from build123d import *

# Parameters (mm, degrees)
F0_W     = 50.8
F0_H     = 54.61
F0_R     = 1.5875
F1_DEPTH = 50.8
F2_R     = 3.96875
F3_DEPTH = 54.611
F4_W     = 50.8
F4_H     = 50.546
F5_DEPTH = 33.9065
F6_W     = 11.43125
F6_H     = 2.032
F7_DEPTH = 2.033


with BuildPart() as f1:
    # F0 (on Front) → F1 (new body)
    with BuildSketch(Plane.XZ):
        Rectangle(F0_W, F0_H)
        with Locations((-9.525, -19.05)):
            Circle(F0_R, mode=Mode.SUBTRACT)
        with Locations((9.525, -19.05)):
            Circle(F0_R, mode=Mode.SUBTRACT)
        with Locations((-9.525, 19.05)):
            Circle(F0_R, mode=Mode.SUBTRACT)
        with Locations((9.525, 19.05)):
            Circle(F0_R, mode=Mode.SUBTRACT)
    extrude(amount=F1_DEPTH)

    # F2 (on face) → F3 (cut, through all)
    with BuildSketch(Plane.XY.offset(27.305)):
        with BuildLine():
            Line((-25.4, -2.032), (-25.4, -50.8))
            Line((-25.4, -50.8), (25.4, -50.8))
            Line((25.4, -50.8), (25.4, -2.032))
            Line((25.4, -2.032), (13.96875, -2.032))
            Line((13.96875, -2.032), (13.96875, -21.96875))
            ThreePointArc((13.96875, -21.96875), (0, -35.9375), (-13.96875, -21.96875))
            Line((-13.96875, -21.96875), (-13.96875, -2.032))
            Line((-13.96875, -2.032), (-25.4, -2.032))
        make_face()
        with Locations((0, -21.96875)):
            Circle(F2_R)
    extrude(amount=-F3_DEPTH, mode=Mode.SUBTRACT)

    # F4 (on face) → F5 (cut, through all)
    with BuildSketch(Plane.XZ.offset(2.032)):
        Rectangle(F4_W, F4_H)
    extrude(amount=F5_DEPTH, mode=Mode.SUBTRACT)

    # F6 (on face) → F7 (cut, through all)
    with BuildSketch(Plane.XZ.offset(2.032)):
        with Locations((-19.684375, 26.289)):
            Rectangle(F6_W, F6_H)
        with Locations((19.684375, 26.289)):
            Rectangle(F6_W, F6_H)
        with Locations((19.684375, -26.289)):
            Rectangle(F6_W, F6_H)
        with Locations((-19.684375, -26.289)):
            Rectangle(F6_W, F6_H)
    extrude(amount=-F7_DEPTH, mode=Mode.SUBTRACT)


solid = f1.part
Geometry: final body of the model. Coordinates: model frame, mm. A direction names the side the tool comes from. Round coordinates to 2 decimals unless told otherwise and drop trailing zeros. Order: outer loops, then holes, each group sorted by start corner. A loop starts at its lowest first (then second) coordinate and runs counter-clockwise, first axis right, second up. Notation, with made-up numbers: (-9.75, -13.75) -> (9.25, -13.75) arc R21 cw to (9.25, 3.25) -> close; hole circle Ø11 at (18.5, 47). An arc over 180 degrees is marked (long way). Put each result on its own line as item: value. Start each with the question number.
Q1. Reachability of faces 5 (the flat face through (0, -15, 25.273)), 6 (the flat face through (25.4, -1, 0)), 7 (the flat face through (-20, -1, 25.273)) from +Z, -Z, +X, -X, +Y, -Y: full face, straight path, thin tool, end or side. Return the list, or none.
Q2. Line query: probe 1 along X at (y, z) = (-1.55, -19.05); probe 2 along Z at (x, y) = (-4, -3.5) (3 decimals); probe 3 along Y at (x, z) = (0, 26.4). Output: solid intervals per line, ascending.
Q3. Section A-A on z = 19.05. Return the cut outline in (x, y), and give its area (3 significant figures).
Q4. Section C-C on y = -16.5. Return the cut outline in (x, z) (3 decimals), and give its area (3 significant figures).
Q5. Section B-B on x = 0. Return the cut outline in (y, z) (1 decimal), and give its area (3 significant figures).
Q6. Section D-D on x = 9.5. Return the cut outline in (y, z) (3 decimals).
Q7. Pull-direction query (X, two-part tool) for faces 1 (the cylindrical face through (7.94, -1, 19.12)), 2 (the cylindrical face through (-0.86, -25.843, -26.275)), 3 (the flat face through (0, -15, -25.273)), 4 (the cylindrical face through (0.307, -35.934, -26.275)); classes: +X half, -X half, draft (parallel to the pull), parting line (faces both ways), or undercut.
Q8. First-contact query: pin 1 (1 mm diameter, centred on y = -14.5, z = 26.5, fed in from -X); pin 2 (1.6 mm diameter, centred on x = 20.5, y = -1.5, fed in from -Z); pin 3 (0.6 mm diameter, centred on y = -11, z = 27, fed in from +X); pin 4 (7 mm diameter, centred on x = 0, y = -21.97, fed in from +Z). Flat tips, straight axial feed; report the tip coordinate or a pass-through.
Ans:
1. face 5: +X, -X, -Y
1. face 6: +Z, -Z, +X, +Y, -Y
1. face 7: +Z, -X, +Y, -Y
2. probe 1: x = -25.4 to -11.11, -7.94 to 7.94, 11.11 to 25.4
2. probe 2: z = -27.305 to -25.273, 25.273 to 27.305
2. probe 3: y = -35.94 to -25.94, -18 to 0
3. outline: (-25.4, -2.03) -> (-11.11, -2.03) -> (-11.11, 0) -> (-25.4, 0) -> close; (-7.94, -2.03) -> (7.94, -2.03) -> (7.94, 0) -> (-7.94, 0) -> close; (11.11, -2.03) -> (25.4, -2.03) -> (25.4, 0) -> (11.11, 0) -> close
3. area: 90.3 mm2
4. outline: (-13.969, -27.305) -> (13.969, -27.305) -> (13.969, -25.273) -> (-13.969, -25.273) -> close; (-13.969, 25.273) -> (13.969, 25.273) -> (13.969, 27.305) -> (-13.969, 27.305) -> close
4. area: 114 mm2
5. outline: (-35.9, -27.3) -> (-25.9, -27.3) -> (-25.9, -25.3) -> (-35.9, -25.3) -> close; (-35.9, 25.3) -> (-25.9, 25.3) -> (-25.9, 27.3) -> (-35.9, 27.3) -> close; (-18, -27.3) -> (0, -27.3) -> (0, 27.3) -> (-18, 27.3) -> (-18, 25.3) -> (-2, 25.3) -> (-2, -25.3) -> (-18, -25.3) -> close
5. area: 217 mm2
6. outline: (-32.21, -27.305) -> (0, -27.305) -> (0, -20.637) -> (-2.032, -20.637) -> (-2.032, -25.273) -> (-32.21, -25.273) -> close; (-32.21, 25.273) -> (-2.032, 25.273) -> (-2.032, 20.637) -> (0, 20.637) -> (0, 27.305) -> (-32.21, 27.305) -> close; (-2.032, -17.463) -> (0, -17.463) -> (0, 17.463) -> (-2.032, 17.463) -> close
7. face 1: undercut
7. face 2: undercut
7. face 3: draft
7. face 4: parting line
8. pin 1: stops at x = -13.97
8. pin 2: stops at z = -25.27
8. pin 3: stops at x = 13.97
8. pin 4: passes through
